```python
from build123d import *

# Parameters (mm, degrees)
SKETCH_1_R      = 5
SKETCH_1_R_2    = 2.5
EXTRUDE_1_DEPTH = 3


with BuildPart() as part:
    # 스케치1 → 보스-돌출1 (new body)
    # profile 1 of 5: a face of its own
    with BuildSketch(Plane.XY):
        with BuildLine():
            Line((8.866410343, 21.94338903), (4.574998823, 21.94338903))
            Line((4.574998823, 21.94338903), (0, 14.743154306))
            Line((0, 14.743154306), (0, 5))
            ThreePointArc((0, 5), (3.535533906, 3.535533906), (5, 0))
            ThreePointArc((5, 0), (0, -5), (-5, 0))
            Line((-5, 0), (-5, -11.202273073))
            Line((-5, -11.202273073), (-20.162460617, -9.822892201))
            ThreePointArc((-20.162460617, -9.822892201), (-21.623929956, -10.278142815), (-22.335434041, -11.633468491))
            Line((-22.335434041, -11.633468491), (-22.441691139, -12.801470088))
            ThreePointArc((-22.441691139, -12.801470088), (-21.986440525, -14.262939427), (-20.631114849, -14.974443512))
            Line((-20.631114849, -14.974443512), (-7.293133085, -16.187845306))
            ThreePointArc((-7.293133085, -16.187845306), (-8.683000099, -31.29485147), (-3.824169556, -45.666529567))
            ThreePointArc((-3.824169556, -45.666529567), (-0.906566305, -46.354001108), (-0.33095704, -43.412283952))
            ThreePointArc((-0.33095704, -43.412283952), (-3.547402259, -28.784479694), (4.574998823, -16.200967549))
            Line((4.574998823, -16.200967549), (8.3701186, -14.978169718))
            ThreePointArc((8.3701186, -14.978169718), (8.662275884, -14.729272874), (8.69193724, -14.346616734))
            ThreePointArc((8.69193724, -14.346616734), (8.365752146, -12.021808556), (8.866410343, -9.728236855))
            Line((8.866410343, -9.728236855), (8.866410343, 21.94338903))
        make_face()
    # profile 2 of 5: a face of its own
    with BuildSketch(Plane.XY):
        Circle(SKETCH_1_R)
        Circle(SKETCH_1_R_2, mode=Mode.SUBTRACT)
    # profile 3 of 5: a face of its own
    with BuildSketch(Plane.XY):
        with BuildLine():
            ThreePointArc((5, 0), (3.535533906, 3.535533906), (0, 5))
            ThreePointArc((0, 5), (-3.535533906, 3.535533906), (-5, 0))
            ThreePointArc((-5, 0), (0, -5), (5, 0))
        make_face()
        Circle(SKETCH_1_R_2, mode=Mode.SUBTRACT)
    # profile 4 of 5: a face of its own
    with BuildSketch(Plane.XY):
        Polygon((8.866410343, 24.08909479), (6.720704583, 24.08909479), (4.574998823, 21.94338903), (8.866410343, 21.94338903), align=None)
    # profile 5 of 5: a face of its own
    with BuildSketch(Plane.XY):
        with BuildLine():
            Line((8.866410343, 21.94338903), (4.574998823, 21.94338903))
            Line((4.574998823, 21.94338903), (0, 14.743154306))
            Line((0, 14.743154306), (0, 5))
            ThreePointArc((0, 5), (3.535533906, 3.535533906), (5, 0))
            ThreePointArc((5, 0), (0, -5), (-5, 0))
            Line((-5, 0), (-5, -11.202273073))
            Line((-5, -11.202273073), (-20.162460617, -9.822892201))
            ThreePointArc((-20.162460617, -9.822892201), (-21.623929956, -10.278142815), (-22.335434041, -11.633468491))
            Line((-22.335434041, -11.633468491), (-22.441691139, -12.801470088))
            ThreePointArc((-22.441691139, -12.801470088), (-21.986440525, -14.262939427), (-20.631114849, -14.974443512))
            Line((-20.631114849, -14.974443512), (-7.293133085, -16.187845306))
            ThreePointArc((-7.293133085, -16.187845306), (-8.683000099, -31.29485147), (-3.824169556, -45.666529567))
            ThreePointArc((-3.824169556, -45.666529567), (-0.906566305, -46.354001108), (-0.33095704, -43.412283952))
            ThreePointArc((-0.33095704, -43.412283952), (-3.547402259, -28.784479694), (4.574998823, -16.200967549))
            Line((4.574998823, -16.200967549), (8.3701186, -14.978169718))
            ThreePointArc((8.3701186, -14.978169718), (8.662275884, -14.729272874), (8.69193724, -14.346616734))
            ThreePointArc((8.69193724, -14.346616734), (8.365752146, -12.021808556), (8.866410343, -9.728236855))
            Line((8.866410343, -9.728236855), (8.866410343, 21.94338903))
        make_face()
    extrude(amount=EXTRUDE_1_DEPTH)


solid = part.part
```
Geometry check sheet. Reference: the model listing, model coordinates, mm. Give positions to 0.01 mm unless a question says otherwise; leave off trailing zeros. Write each loop counter-clockwise with the first axis right and the second up, starting at its lowest first coordinate (ties: lowest second). Pieces come first, ordered by that corner, then holes. Notation, with made-up numbers: (-38.5, -33.75) - (4.5, -33.75) arc R11 ccw to (4.5, -16.75) - close; hole circle Ø3 at (47.25, 19). An arc over 180 degrees is marked (long way). Use a Markdown table: item, result.
Q1. Go/stop test with flat-tipped pins: P1, Ø2, axis at x = 1.5, y = 4.5, coming from the -Z side; P2, Ø1.5, axis at y = 9, z = 2, coming from the -X side. Record where each tip stops, or that it passes through.
Computed:
| item | result |
|---|---|
| P1 | stops at z = 0 |
| P2 | stops at x = 0 |
Q2. Section check C-C, the plane x = 6. Enter the section's corners in (y, z).
Computed:
| item | result |
|---|---|
| outline | (-15.74, 0) - (23.37, 0) - (23.37, 3) - (-15.74, 3) - close |
Q3. Thickness scan on L1, parallel to X at y = -7, z = 1.75; L2, parallel to X at y = 17, z = 2.05; L3, parallel to Y at x = 6, z = 0.3. Record the ranges inside material, lowest first. Write a range as [from, to].
Computed:
| item | result |
|---|---|
| L1 | x = [-5, 8.87] |
| L2 | x = [1.43, 8.87] |
| L3 | y = [-15.74, 23.37] |
Q4. Draft check along X on faces 1 (the face through (-12.48, -10.52, 1.48)), 2 (the face through (-22, -14.246, 1.479)), 3 (the face through (8.365, -12.055, 1.479)). Enter one of: pulls with the +X half, pulls with the -X half, needs draft (parallel to the pull), parting line crosses it, or undercut.
Computed:
| item | result |
|---|---|
| face 1 | undercut |
| face 2 | pulls with the -X half |
| face 3 | pulls with the +X half |
Q5. Section check B-B, the plane y = -6. Enter the section's corners in (x, z).
Computed:
| item | result |
|---|---|
| outline | (-5, 0) - (8.87, 0) - (8.87, 3) - (-5, 3) - close |
Q6. Section check A-A, the plane z = 2.3. Enter the section's corners in (x, y) (3 decimals).
Computed:
| item | result |
|---|---|
| outline | (-22.442, -12.801) arc R2 ccw to (-20.631, -14.974) - (-7.293, -16.188) arc R36.58 ccw to (-3.824, -45.667) arc R2.08 ccw (long way) to (-0.331, -43.412) arc R19.469 cw to (4.575, -16.201) - (8.37, -14.978) arc R0.5 ccw to (8.692, -14.347) arc R6.661 cw to (8.866, -9.728) - (8.866, 24.089) - (6.721, 24.089) - (4.575, 21.943) - (0, 14.743) - (0, 5) arc R5 ccw to (-5, 0) - (-5, -11.202) - (-20.162, -9.823) arc R2 ccw to (-22.335, -11.633) - close; hole circle Ø5 at (0, 0) |
